Part model, mm, in its own coordinate system. Face numbers are marked on the shaded views. A direction names the side the tool comes from. Give positions to 0.01 mm unless a question says otherwise; leave off trailing zeros. Loops run counter-clockwise (first coordinate to the right, second up) from the corner with the lowest first, then second, coordinate; pieces in that order, holes last. Notation, with made-up numbers: M 40,-1.75 L 72,-1.75 A20 cw 72,3.25 Z; hole C 49,4.25 d2. An arc over 180 degrees is marked long. Answer in a Markdown table with one row per item.
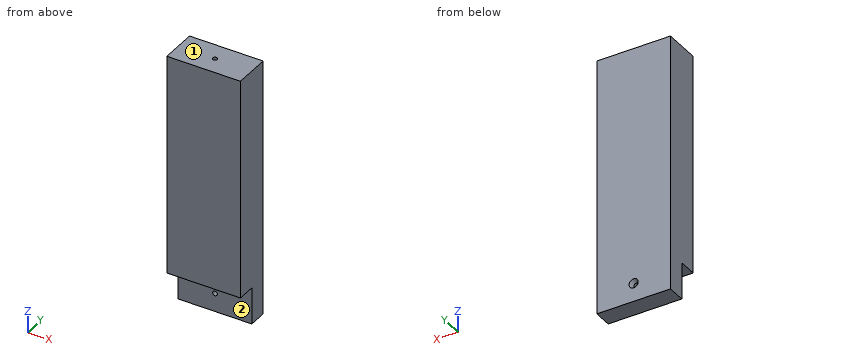
from build123d import *

# Parameters (mm, degrees)
F0_W     = 101.6
F0_H     = 50.8
F1_DEPTH = 355.6
F2_W     = 101.6
F2_H     = 25.4
F3_DEPTH = 50.8
F4_R     = 3.175
F5_DEPTH = 50.801
F6_R     = 3.175
F7_DEPTH = 25.4
F8_R     = 6.35
F9_DEPTH = 6.35
F9_TAPER = 30


with BuildPart() as f1:
    # F0 (on Top) → F1 (new body)
    with BuildSketch(Plane.XY):
        Rectangle(F0_W, F0_H)
    extrude(amount=F1_DEPTH)

    # F2 (on face) → F3 (cut)
    with BuildSketch(Plane(origin=(0, 0, 0), x_dir=(1, 0, 0), z_dir=(0, 0, -1))):
        with Locations((0, 12.7)):
            Rectangle(F2_W, F2_H)
    extrude(amount=-F3_DEPTH, mode=Mode.SUBTRACT)

    # F4 (on face) → F5 (cut, through all)
    with BuildSketch(Plane(origin=(0, 25.4, 0), x_dir=(-1, 0, 0), z_dir=(0, 1, 0))):
        with Locations((0, 25.4)):
            Circle(F4_R)
    extrude(amount=-F5_DEPTH, mode=Mode.SUBTRACT)

    # F6 (on face) → F7 (cut)
    with BuildSketch(Plane.XY.offset(355.6)):
        Circle(F6_R)
    extrude(amount=-F7_DEPTH, mode=Mode.SUBTRACT)

    # F8 (on face) → F9 (cut)
    with BuildSketch(Plane(origin=(0, 25.4, 0), x_dir=(-1, 0, 0), z_dir=(0, 1, 0))):
        with Locations((0, 25.4)):
            Circle(F8_R)
    extrude(amount=-F9_DEPTH, taper=F9_TAPER, mode=Mode.SUBTRACT)


solid = f1.part
(1) Pin check, flat tip, straight feed: pin 1 Ø8.5 at (x, z) = (0, 25.4) entering from -Y. Stop position of the tip, or through.
Recorded:
| item | result |
|---|---|
| pin 1 | stops at y = 0 |
(2) Which spindle directions (+Z, -Z, +X, -X, +Y, -Y) get a long thin tool onto all of the face, cutting with end or side? Do the marked faces 1 and 2. Say none if no direction does.
Recorded:
| item | result |
|---|---|
| face 1 | +Z, +X, -X, +Y, -Y |
| face 2 | -Z, +X, -X, -Y |
(3) Drill centre lines: line 1 along X through (y, z) = (11, 25); line 2 along Y through (x, z) = (0, 346) (3 decimals); line 3 along Z through (x, y) = (0, 5.25) (3 decimals). Where is each one in solid material? Low to high.
Recorded:
| item | result |
|---|---|
| line 1 | x = -50.8 to -3.15, 3.15 to 50.8 |
| line 2 | y = -25.4 to -3.175, 3.175 to 25.4 |
| line 3 | z = 0 to 22.225, 28.575 to 355.6 |
(4) Saw through at A-A (x = 0). Write the cut outline in (y, z) (3 decimals), plus the area to 3 significant figures.
Recorded:
| item | result |
|---|---|
| outline | M -25.4,50.8 L 0,50.8 L 0,28.575 L 19.901,28.575 L 25.4,31.75 L 25.4,355.6 L 3.175,355.6 L 3.175,330.2 L -3.175,330.2 L -3.175,355.6 L -25.4,355.6 Z; M 0,0 L 25.4,0 L 25.4,19.05 L 19.901,22.225 L 0,22.225 Z |
| area | 16,400 mm^2 |
(5) Saw through at C-C (y = -20). Write the cut outline in (x, z).
Recorded:
| item | result |
|---|---|
| outline | M -50.8,50.8 L 50.8,50.8 L 50.8,355.6 L -50.8,355.6 Z |
(6) Saw through at B-B (x = 24). Write the cut outline in (y, z).
Recorded:
| item | result |
|---|---|
| outline | M -25.4,50.8 L 0,50.8 L 0,0 L 25.4,0 L 25.4,355.6 L -25.4,355.6 Z |
